Check sheet for the modelled part. Datum: model origin and axes. Units: mm. Face numbers are marked on the shaded views. A direction names the side the tool comes from. Coordinates: 2 decimals unless noted, no trailing zeros. One line per item, written item: value. Start each with the question number.
1) Set-up check for the marked faces 3 and 4: record each of +Z, -Z, +X, -X, +Y, -Y from which the full face is reachable in a straight line by a thin tool's end or side.
2) Draft check along Z on the marked faces 1 and 2. Enter one of: +Z half, -Z half, draft (parallel to the pull), parting line (faces both ways), or undercut.
3) Gauge pin test, flat ends, axial feed: P1, Ø8, axis at x = -13, y = 91, coming from the +Z side; P2, Ø1.5, axis at y = 79, z = -8, coming from the -X side; P3, Ø10, axis at x = -10, y = 98.5, coming from the +Z side. Record the tip position at first contact, or that the pin passes through.
4) Scan lines: line 1 along Z through (x, y) = (-13, 86); line 2 along X through (y, z) = (58.5, 6); line 3 along Z through (x, y) = (-7, 92). Record each from-to range of solid material in increasing order. Write a range as [from, to].
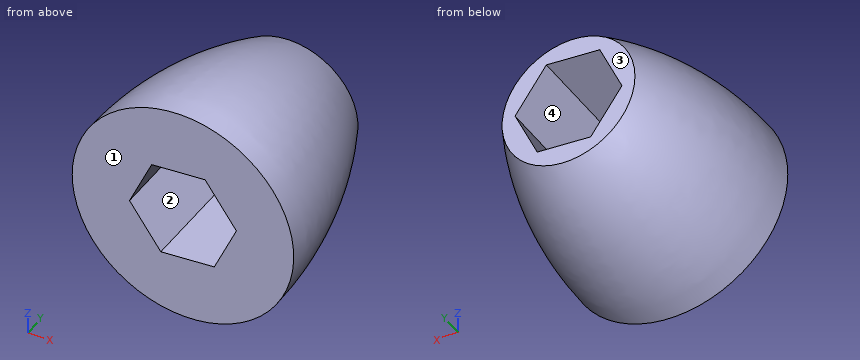
```python
from build123d import *

# Parameters (mm, degrees)
SKETCH1_R               = 19.05
BOSS_EXTRUDE1_DEPTH     = 104.775
CUT_EXTRUDE1_DEPTH      = 104.775
SKETCH5_W               = 79.059329342
SKETCH5_H               = 52.3875
CUT_EXTRUDE2_DEPTH      = 32.7500001
CUT_EXTRUDE2_DEPTH_BACK = 32.7500001


with BuildPart() as part:
    # Sketch1 → Boss-Extrude1 (new body)
    with BuildSketch(Plane(origin=(0, 0, 0), x_dir=(1, 0, 0), z_dir=(0, 1, 0))):
        Circle(SKETCH1_R)
    extrude(amount=BOSS_EXTRUDE1_DEPTH)

    # Sketch2 → Cut-Extrude1 (cut)
    with BuildSketch(Plane.XZ):
        Polygon((-15.323636661, -1.510781079), (-6.353443536, -14.026049167), (8.970193125, -12.515268087), (15.323636661, 1.510781079), (6.353443536, 14.026049167), (-8.970193125, 12.515268087), align=None)
    extrude(amount=-CUT_EXTRUDE1_DEPTH, mode=Mode.SUBTRACT)

    # Sketch4 → Revolve1 (revolve)
    with BuildSketch(Plane.XY):
        with BuildLine():
            Line((-19.05, 104.775), (-19.05, 0))
            ThreePointArc((-19.05, 0), (-31.75, 52.3875), (-19.05, 104.775))
        make_face()
    revolve(axis=Axis((0, 0, 0), (0, 1, 0)))

    # Sketch5 → Cut-Extrude2 (cut, two sides)
    with BuildSketch(Plane.XY) as cut_extrude2_sk:
        with Locations((-0.139680794, 26.19375)):
            Rectangle(SKETCH5_W, SKETCH5_H)
    extrude(amount=CUT_EXTRUDE2_DEPTH, mode=Mode.SUBTRACT)
    extrude(cut_extrude2_sk.sketch, amount=-CUT_EXTRUDE2_DEPTH_BACK, mode=Mode.SUBTRACT)


solid = part.part
```
Answers:
1. face 3: +Z, -Z, +X, -X, +Y
1. face 4: +Y, -Y
2. face 1: draft
2. face 2: undercut
3. P1: stops at z = 23.94
3. P2: stops at x = -27.75
3. P3: stops at z = 22.66
4. line 1: z = [-23.32, -4.75], [3.62, 23.32]
4. line 2: x = [-31.01, -11.92], [12.11, 31.01]
4. line 3: z = [-23.66, -13.12], [12.71, 23.66]
